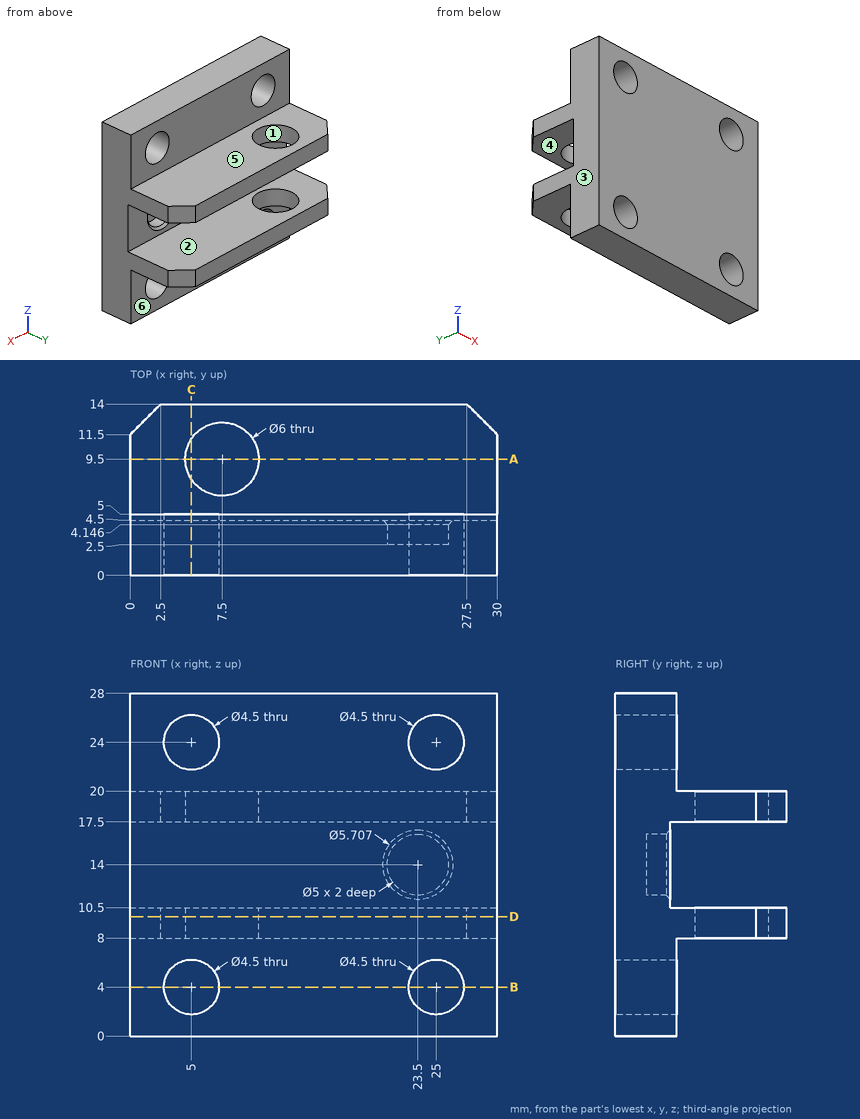
Design review of the part shown in the three views and the two pictorial views. Dimensions are in mm from the part's minimum x, y and z. A direction names the side the tool comes from. Give positions to 0.01 mm unless a question says otherwise; leave off trailing zeros. Write each loop counter-clockwise with the first axis right and the second up, starting at its lowest first coordinate (ties: lowest second). Pieces come first, ordered by that corner, then holes.
(1) Add section B-B (z = 4). Give the boundary of the cut face in (x, y), and give its area (3 significant figures).
Checked values:
outline: (0, 0) - (2.75, 0) - (2.75, 5) - (0, 5) - close; (7.25, 0) - (22.75, 0) - (22.75, 5) - (7.25, 5) - close; (27.25, 0) - (30, 0) - (30, 5) - (27.25, 5) - close
area: 105 mm2
(2) Mouldability with a two-part tool opening along X and no side actions: class the marked faces 1, 2 and 3 as +X half, -X half, draft (parallel to the pull), parting line (faces both ways), or undercut.
Checked values:
face 1: undercut
face 2: draft
face 3: -X half
(3) Tool access review of the marked faces 4, 5 and 6: name each direction out of +Z, -Z, +X, -X, +Y, -Y from which nothing blocks a thin tool from reaching the whole face with its end or side.
Checked values:
face 4: +X, -X, +Y
face 5: +Z, +X, -X, +Y
face 6: -Z, +X, -X, +Y
(4) Wall thickness on line 1 along X through (y, z) = (2.2, 4); line 2 along Z through (x, y) = (24.25, 3.25) (1 decimal); line 3 along Z through (x, y) = (25, 8): over which ranges is each line inside the solid? List them lowest first.
Checked values:
line 1: x = 0 to 2.75, 7.25 to 22.75, 27.25 to 30
line 2: z = 0 to 1.9, 6.1 to 11.6, 16.4 to 21.9, 26.1 to 28
line 3: z = 8 to 10.5, 17.5 to 20
(5) Clearance check with flat-ended pins moving along their axes: pin 1 Ø4 at (x, z) = (5, 24) entering from +Y; pin 2 Ø6 at (x, z) = (25, 4) entering from +Y; pin 3 Ø5 at (x, y) = (17, 8.5) entering from +Z; pin 4 Ø1.5 at (x, z) = (24, 13.5) entering from +Y. State where each tip first meets the part, or that it passes through.
Checked values:
pin 1: passes through
pin 2: stops at y = 5
pin 3: stops at z = 20
pin 4: stops at y = 2.5
(6) Add section C-C (x = 5). Give the boundary of the cut face in (y, z).
Checked values:
outline: (0, 0) - (5, 0) - (5, 1.75) - (0, 1.75) - close; (0, 6.25) - (5, 6.25) - (5, 8) - (7.84, 8) - (7.84, 10.5) - (4.5, 10.5) - (4.5, 17.5) - (7.84, 17.5) - (7.84, 20) - (5, 20) - (5, 21.75) - (0, 21.75) - close; (0, 26.25) - (5, 26.25) - (5, 28) - (0, 28) - close; (11.16, 8) - (14, 8) - (14, 10.5) - (11.16, 10.5) - close; (11.16, 17.5) - (14, 17.5) - (14, 20) - (11.16, 20) - close
(7) Add section D-D (z = 9.75). Give the boundary of the cut face in (x, y).
Checked values:
outline: (0, 0) - (30, 0) - (30, 11.5) - (27.5, 14) - (2.5, 14) - (0, 11.5) - close; hole circle Ø6 at (7.5, 9.5)
(8) Add section A-A (y = 9.5). Give the boundary of the cut face in (x, z), and give its area (3 significant figures).
Checked values:
outline: (0, 8) - (4.5, 8) - (4.5, 10.5) - (0, 10.5) - close; (0, 17.5) - (4.5, 17.5) - (4.5, 20) - (0, 20) - close; (10.5, 8) - (30, 8) - (30, 10.5) - (10.5, 10.5) - close; (10.5, 17.5) - (30, 17.5) - (30, 20) - (10.5, 20) - close
area: 120 mm2
